from build123d import *

# Parameters (mm, degrees)
SKETCH1_R           = 12.5
BOSS_EXTRUDE1_DEPTH = 6
BOSS_EXTRUDE2_DEPTH = 6
FILLET1_R           = 5


with BuildPart() as part:
    # Sketch1 → Boss-Extrude1 (new body)
    with BuildSketch(Plane.XY):
        with BuildLine():
            Line((-22.5, 0), (-22.5, -30))
            Line((-22.5, -30), (-6.707199182, -30))
            Line((-6.707199182, -30), (-6.707199182, -24))
            Line((-6.707199182, -24), (6.707199182, -24))
            Line((6.707199182, -24), (6.707199182, -30))
            Line((6.707199182, -30), (22.5, -30))
            Line((22.5, -30), (22.5, 0))
            ThreePointArc((22.5, 0), (0, 22.5), (-22.5, 0))
        make_face()
        Circle(SKETCH1_R, mode=Mode.SUBTRACT)
    extrude(amount=BOSS_EXTRUDE1_DEPTH)

    # Sketch2 → Boss-Extrude2 (add)
    with BuildSketch(Plane.XY):
        Polygon((-22.5, -30), (-26, -30), (-26, -16.5), (-24, -16.5), (-24, -11.5), (-26, -11.5), (-26, -6), (-31, -6), (-31, -11.5), (-33, -11.5), (-33, -16.5), (-31, -16.5), (-31, -30), (-34.5, -30), (-34.5, 0), (-22.5, 0), align=None)
    boss_extrude2 = extrude(amount=BOSS_EXTRUDE2_DEPTH)

    # Mirror1: Boss-Extrude2 across plane
    add(boss_extrude2.mirror(Plane(origin=(0, 0, 0), x_dir=(0, 0, 1), z_dir=(1, 0, 0))))

    # Fillet1
    fillet1_edges = [part.edges().sort_by_distance(p)[0] for p in [
        (22.5, 0, 3),
        (-22.5, 0, 3),
        (-34.5, 0, 3),
        (34.5, 0, 3),
    ]]
    fillet(fillet1_edges, radius=FILLET1_R)


solid = part.part
Design review of the part built by this model. Coordinates are the model's own, in mm. A direction names the side the tool comes from. Round coordinates to 2 decimals unless told otherwise and drop trailing zeros. Loops run counter-clockwise (first coordinate to the right, second up) from the corner with the lowest first, then second, coordinate; pieces in that order, holes last. Notation, with made-up numbers: M -5,-27 L 11,-27 A24 cw 11,-13 Z; hole C 24,21.5 d9. An arc over 180 degrees is marked long. Answer as a JSON object with one key per item and string values.
Item 1: We need section B-B on y = -14. Give the boundary of the cut face in (x, z).
Answer sheet:
{"outline": "M -34.5,0 L -33,0 L -33,6 L -34.5,6 Z; M -24,0 L 24,0 L 24,6 L -24,6 Z; M 33,0 L 34.5,0 L 34.5,6 L 33,6 Z"}
Item 2: The part is to be moulded in two halves that separate along X. For faces 4 (the flat face through (0, -15, 0)), 5 (the flat face through (6.707, -27, 3)), 6 (the cylindrical face through (23.806, 1.188, 3.042)), say which applies: pulls with the +X half, pulls with the -X half, needs draft (parallel to the pull), parting line crosses it, or undercut.
Answer sheet:
{"face 4": "needs draft", "face 5": "undercut", "face 6": "pulls with the +X half"}
Item 3: Machinability: for faces 1 (the flat face through (32, -11.5, 3)), 2 (the flat face through (28, 0, 3)), 3 (the flat face through (26, -9, 3)), which of the approach directions +Z, -Z, +X, -X, +Y, -Y give a long, thin tool a straight path to every point of the face, cutting with its end or side? Answer none if there is none.
Answer sheet:
{"face 1": "+Z, -Z", "face 2": "+Z, -Z, +X, +Y", "face 3": "+Z, -Z, -Y"}
Item 4: Wall thickness on L1, parallel to X at y = -14, z = 2.2; L2, parallel to X at y = -8, z = 1.8; L3, parallel to Y at x = 0, z = 3.2: over which ranges is each line inside the solid? List them lowest first. Write a range as from..to.
Answer sheet:
{"L1": "x = -34.5..-33, -24..24, 33..34.5", "L2": "x = -34.5..-31, -26..-9.6, 9.6..26, 31..34.5", "L3": "y = -24..-12.5, 12.5..22.5"}
Item 5: We need section C-C on y = -3.5. Give the boundary of the cut face in (x, z).
Answer sheet:
{"outline": "M -34.27,0 L -12,0 L -12,6 L -34.27,6 Z; M 12,0 L 34.27,0 L 34.27,6 L 12,6 Z"}
Item 6: We need section D-D on y = 13.5. Give the boundary of the cut face in (x, z).
Answer sheet:
{"outline": "M -18,0 L 18,0 L 18,6 L -18,6 Z"}
Item 7: We need section A-A on x = 0. Give the boundary of the cut face in (y, z), and give its area (3 significant figures).
Answer sheet:
{"outline": "M -24,0 L -12.5,0 L -12.5,6 L -24,6 Z; M 12.5,0 L 22.5,0 L 22.5,6 L 12.5,6 Z", "area": "129 mm^2"}
Item 8: Clearance check with flat-ended pins moving along their axes: P1, Ø0.6, axis at x = 32.5, z = 4, coming from the +Y side; P2, Ø1.5, axis at x = 29.5, z = 3, coming from the -Y side; P3, Ø10, axis at x = 11.5, y = 4, coming from the -Z side; P4, Ø1.6, axis at x = -31.5, z = 2, coming from the +Y side. State where each tip first meets the part, or that it passes through.
Answer sheet:
{"P1": "stops at y = -0.79", "P2": "stops at y = -6", "P3": "stops at z = 0", "P4": "stops at y = -0.15"}
